Autodesk Inventor part; units mm, degrees
ref_plane "YZ Plane" through (0, 0, 0) normal (1, 0, 0) x (0, 1, 0)
ref_plane "XZ Plane" through (0, 0, 0) normal (0, 1, 0) x (-1, 0, 0)
ref_plane "XY Plane" through (0, 0, 0) normal (0, 0, 1) x (1, 0, 0)
sketch "Sketch1" plane through (0, 0, 0) normal (0, 1, 0) x (-1, 0, 0)
  line L0 (-59.7535, -47.0027) -> (59.7535, -47.0027)
  line L1 (59.7535, -47.0027) -> (59.7535, 47.0027)
  line L2 (59.7535, 47.0027) -> (-59.7535, 47.0027)
  line L3 (-59.7535, 47.0027) -> (-59.7535, -47.0027)
  line L4 (-59.7535, -47.0027) -> (59.7535, 47.0027) construction
  line L5 (59.7535, -47.0027) -> (-59.7535, 47.0027) construction
  point P0 (0, 0)
  dimension "d0" = 119.507
  dimension "d1" = 94.0054
extrude "Extrusion1" add sketch "Sketch1" along normal mid plane 2.2606
sketch "Sketch2" plane through (0, 1.1303, 0) normal (0, 1, 0) x (1, 0, 0)
  line L0 (-59.7535, 47.0027) -> (-59.7535, -47.0027)
  line L1 (59.7535, -47.0027) -> (59.7535, 47.0027)
  line L2 (-59.7535, -47.0027) -> (59.7535, -47.0027)
  line L3 (59.7535, -47.0027) -> (59.7535, 47.0027)
  line L4 (59.7535, 47.0027) -> (-59.7535, 47.0027)
  line L5 (-59.7535, 47.0027) -> (-59.7535, -47.0027)
  line L6 (57.4929, -44.7421) -> (-57.4929, 44.7421) construction
  line L7 (-57.4929, -44.7421) -> (57.4929, 44.7421) construction
  line L8 (-59.7535, -47.0027) -> (59.7535, -47.0027)
  line L9 (-59.7535, -47.0027) -> (-50.7619, -47.0027)
  line L10 (-59.7535, -38.0111) -> (-59.7535, -47.0027)
  line L11 (-59.7535, 47.0027) -> (-50.7619, 47.0027)
  line L12 (-59.7535, 38.0111) -> (-59.7535, 47.0027)
  line L13 (59.7535, 47.0027) -> (-59.7535, 47.0027)
  line L14 (59.7535, 47.0027) -> (50.7619, 47.0027)
  line L15 (59.7535, 38.0111) -> (59.7535, 47.0027)
  line L16 (59.7535, -47.0027) -> (50.7619, -47.0027)
  line L17 (59.7535, -38.0111) -> (59.7535, -47.0027)
  line L18 (-50.7619, -44.7421) -> (-50.7619, -38.0111)
  line L19 (-50.7619, -38.0111) -> (-57.4929, -38.0111)
  line L20 (-57.4929, 38.0111) -> (-50.7619, 38.0111)
  line L21 (-50.7619, 38.0111) -> (-50.7619, 44.7421)
  line L22 (50.7619, 38.0111) -> (57.4929, 38.0111)
  line L23 (50.7619, 44.7421) -> (50.7619, 38.0111)
  line L24 (57.4929, -38.0111) -> (50.7619, -38.0111)
  line L25 (50.7619, -38.0111) -> (50.7619, -44.7421)
  line L26 (-50.7619, -44.7421) -> (50.7619, -44.7421)
  line L27 (57.4929, -38.0111) -> (57.4929, 38.0111)
  line L28 (50.7619, 44.7421) -> (-50.7619, 44.7421)
  line L29 (-57.4929, 38.0111) -> (-57.4929, -38.0111)
  point P0 (0, 0)
  dimension "d4" = 114.9858
  dimension "d5" = 89.4842
  dimension "d6" = 8.9916
  dimension "d7" = 8.9916
  dimension "d10" = 8.9916
  dimension "d11" = 8.9916
extrude "Extrusion2" add sketch "Sketch2" along normal blind 38.1
sketch "Sketch3" plane through (0, 1.1303, 0) normal (0, 1, 0) x (1, 0, 0)
  circle A0 centre (0, -25.4) radius 2.0828
  circle A1 centre (0, 25.4) radius 2.0828
  point P0 (0, 0)
  dimension "d18" = 4.1656
  dimension "d19" = 4.1656
extrude "Extrusion3" cut sketch "Sketch3" against normal through all
sketch "Sketch7" plane through (0, 1.1303, 0) normal (0, 1, 0) x (1, 0, 0)
  line L0 (32.9946, -9.9949) -> (-32.9946, 9.9949) construction
  line L1 (-32.9946, -9.9949) -> (32.9946, 9.9949) construction
  circle A0 centre (-32.9946, -9.9949) radius 1.4986
  circle A1 centre (-32.9946, 9.9949) radius 1.4986
  circle A2 centre (32.9946, 9.9949) radius 1.4986
  circle A3 centre (32.9946, -9.9949) radius 1.4986
  line L2 (47.498, -29.9974) -> (-47.498, 29.9974) construction
  line L3 (-47.498, -29.9974) -> (47.498, 29.9974) construction
  line L4 (-47.498, 29.9974) -> (-41.148, 29.9974) construction
  line L5 (47.498, 29.9974) -> (53.848, 29.9974) construction
  line L6 (47.2281, 30.3609) -> (-47.2281, 30.3609)
  line L7 (-47.2281, -30.3609) -> (47.2281, -30.3609)
  line L8 (47.2281, -30.3609) -> (47.2281, 30.3609)
  line L9 (47.2281, 30.3609) -> (-47.2281, -30.3609) construction
  line L10 (-47.2281, 30.3609) -> (47.2281, -30.3609) construction
  line L11 (-47.2568, -30.3794) -> (-46.2408, -30.3794)
  line L12 (-46.2408, -29.3634) -> (-47.2568, -29.3634)
  line L13 (-47.2568, -29.3634) -> (-47.2568, -30.3794)
  line L14 (-47.2281, 30.3609) -> (-46.2121, 30.3609)
  line L15 (-46.2121, 29.3449) -> (-47.2281, 29.3449)
  line L16 (-47.2281, 29.3449) -> (-47.2281, 30.3609)
  line L17 (47.2281, 30.3609) -> (46.2121, 30.3609)
  line L18 (46.2121, 29.3449) -> (47.2281, 29.3449)
  line L19 (47.2281, 29.3449) -> (47.2281, 30.3609)
  line L20 (47.2281, -30.3609) -> (46.2121, -30.3609)
  line L21 (46.2121, -29.3449) -> (47.2281, -29.3449)
  line L22 (47.2281, -29.3449) -> (47.2281, -30.3609)
  circle A4 centre (46.2121, -29.3449) radius 1.524
  circle A5 centre (46.2121, 29.3449) radius 1.524
  circle A6 centre (-46.2121, 29.3449) radius 1.524
  circle A7 centre (-46.2408, -29.3634) radius 1.524
  point P0 (0, 0)
  dimension "d48" = 19.9898
  dimension "d49" = 2.9972
  dimension "d50" = 2.9972
  dimension "d51" = 2.9972
  dimension "d52" = 2.9972
  dimension "d78" = 94.4562
  dimension "d79" = 60.7219
  dimension "d80" = 1.016
  dimension "d81" = 1.016
  dimension "d82" = 1.016
  dimension "d83" = 1.016
  dimension "d84" = 1.016
  dimension "d85" = 1.016
  dimension "d86" = 1.016
  dimension "d87" = 1.016
  dimension "d88" = 3.048
  dimension "d89" = 3.048
  dimension "d90" = 3.048
  dimension "d91" = 3.048
sketch "Sketch8" plane through (50.7619, 1.1303, 44.7421) normal (0, 0, -1) x (-1, 0, 0)
  circle A0 centre (23.9014, 19.05) radius 3.175
  circle A1 centre (38.989, 19.05) radius 3.175
  point P0 (50.7619, -1.1303)
  dimension "d74" = 6.35
  dimension "d75" = 6.35
extrude "Extrusion7" cut sketch "Sketch8" against normal through all
extrude "Extrusion8" cut sketch "Sketch7" against normal through all
properties part number "546-1590BBS-ADF4360-9"
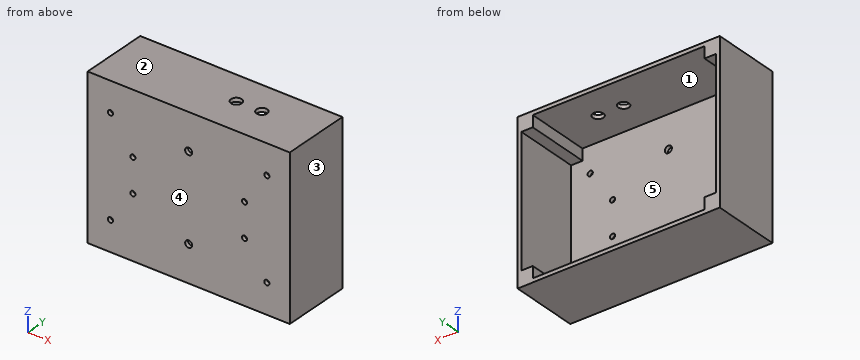
Can you work these out from the model? Positions are in its coordinate system, mm. Face numbers are marked on the shaded views. A direction names the side the tool comes from. Coordinates: 2 decimals unless noted, no trailing zeros. Loops run counter-clockwise (first coordinate to the right, second up) from the corner with the lowest first, then second, coordinate; pieces in that order, holes last.
1) Imagine slicing it at A-A on x = 0. List the corners of the cut face in (y, z) for me.
2) Imagine slicing it at B-B on y = 10.5. List the corners of the cut face in (x, z) for me, plus the area to 3 significant figures.
3) Thinking about a two-plate mould opening in X: for the marked faces 3, 4 and 5, which applies, pulls with the +X half, pulls with the -X half, needs draft (parallel to the pull), parting line crosses it, or undercut?
4) Which directions (+Z, -Z, +X, -X, +Y, -Y) give clear straight access to the entire face, cutting with the end or side of a thin tool? Please do the marked faces 1 and 2.
5) Imagine slicing it at D-D on z = -6. List the corners of the cut face in (x, y) for me.
6) I need wall thicknesses on probe 1 along Z at (x, y) = (-36.5, 27); probe 2 along X at (y, z) = (17, -27.5); probe 3 along Y at (x, z) = (41.5, 32.5). Which ranges of each line are inside material? Lowest first, please.
7) Imagine slicing it at C-C on z = 25.4. List the corners of the cut face in (x, y) for me, plus the area to 3 significant figures.
8) For pin 1 (1 mm diameter, centred on x = 25.5, z = 34, fed in from +Y); pin 2 (5 mm diameter, centred on x = 11.77, y = 20.18, fed in from +Z), each with a flat end and sliding along its axis, tell me the tip position at first contact or that it passes through.
Completed:
1. outline: (-1.13, -47) - (39.23, -47) - (39.23, -44.74) - (1.13, -44.74) - (1.13, -27.48) - (-1.13, -27.48) - close; (-1.13, -23.32) - (1.13, -23.32) - (1.13, 23.32) - (-1.13, 23.32) - close; (-1.13, 27.48) - (1.13, 27.48) - (1.13, 44.74) - (39.23, 44.74) - (39.23, 47) - (-1.13, 47) - close
2. outline: (-59.75, -47) - (59.75, -47) - (59.75, 47) - (-59.75, 47) - close; hole (-57.49, -38.01) - (-50.76, -38.01) - (-50.76, -44.74) - (50.76, -44.74) - (50.76, -38.01) - (57.49, -38.01) - (57.49, 38.01) - (50.76, 38.01) - (50.76, 44.74) - (-50.76, 44.74) - (-50.76, 38.01) - (-57.49, 38.01) - close
2. area: 1,130 mm2
3. face 3: pulls with the +X half
3. face 4: needs draft
3. face 5: undercut
4. face 1: +Y
4. face 2: +Z, +X, -X, +Y, -Y
5. outline: (-59.75, -1.13) - (59.75, -1.13) - (59.75, 39.23) - (57.49, 39.23) - (57.49, 1.13) - (-57.49, 1.13) - (-57.49, 39.23) - (-59.75, 39.23) - close
6. probe 1: z = -47 to -44.74, 44.74 to 47
6. probe 2: x = -59.75 to -57.49, 57.49 to 59.75
6. probe 3: y = -1.13 to 1.13
7. outline: (-59.75, -1.13) - (-2.08, -1.13) - (-2.08, 1.13) - (-57.49, 1.13) - (-57.49, 39.23) - (-59.75, 39.23) - close; (2.08, -1.13) - (59.75, -1.13) - (59.75, 39.23) - (57.49, 39.23) - (57.49, 1.13) - (2.08, 1.13) - close
7. area: 433 mm2
8. pin 1: stops at y = 1.13
8. pin 2: stops at z = -44.74
